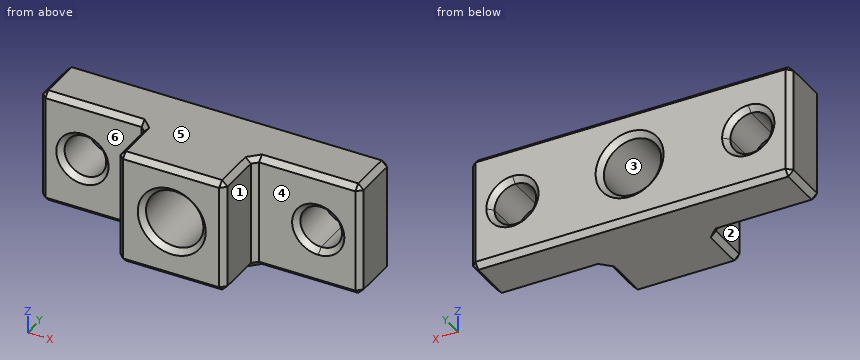
```python
from build123d import *

# Parameters (mm, degrees)
F0_W      = 30.2609670907
F0_H      = 10.7729053125
F1_DEPTH  = 10
F2_W      = 10.0509477779
F2_H      = 10.7729053125
F3_DEPTH  = 5
F4_W      = 10.0912228227
F4_H      = 10.7729053125
F5_DEPTH  = 5
F6_W      = 10.084872134
F6_H      = 10.7729053125
F7_DEPTH  = 5
F8_R      = 2.7105464677
F9_DEPTH  = 25
F11_DEPTH = 25
F13_DEPTH = 25
F14_SIZE  = 0.5


with BuildPart() as f1:
    # F0 (on Front) → F1 (new body)
    with BuildSketch(Plane.XZ):
        with Locations((15.1304835454, -5.3864526562)):
            Rectangle(F0_W, F0_H)
    extrude(amount=F1_DEPTH)

    # F2 (on face) → F3 (join)
    with BuildSketch(Plane.XZ.offset(10)):
        with Locations((5.025473889, -5.3864526562)):
            Rectangle(F2_W, F2_H)
    extrude(amount=-F3_DEPTH)

    # F4 (on face) → F5 (cut)
    with BuildSketch(Plane.XZ.offset(10)):
        with Locations((5.0456114113, -5.3864526562)):
            Rectangle(F4_W, F4_H)
    extrude(amount=-F5_DEPTH, mode=Mode.SUBTRACT)

    # F6 (on face) → F7 (cut)
    with BuildSketch(Plane.XZ.offset(10)):
        with Locations((25.2185310237, -5.3864526562)):
            Rectangle(F6_W, F6_H)
    extrude(amount=-F7_DEPTH, mode=Mode.SUBTRACT)

    # F8 (on face) → F9 (cut)
    with BuildSketch(Plane.XZ.offset(10)):
        with Locations((15.200487338, -5.2238842472)):
            Circle(F8_R)
    extrude(amount=-F9_DEPTH, mode=Mode.SUBTRACT)

    # F10 (on face) → F11 (cut)
    with BuildSketch(Plane.XZ.offset(5)):
        with BuildLine():
            ThreePointArc((5.9674986844, -5.3864526562), (5.3912316617, -3.9952209945), (4, -3.4189539719))
            Line((4, -3.4189539719), (4, -7.3539513406))
            ThreePointArc((4, -7.3539513406), (5.3912316617, -6.7776843179), (5.9674986844, -5.3864526562))
        make_face()
        with BuildLine():
            Line((4, -7.3539513406), (4, -3.4189539719))
            ThreePointArc((4, -3.4189539719), (2.0325013156, -5.3864526562), (4, -7.3539513406))
        make_face()
    extrude(amount=-F11_DEPTH, mode=Mode.SUBTRACT)

    # F12 (on face) → F13 (cut)
    with BuildSketch(Plane.XZ.offset(5)):
        with BuildLine():
            ThreePointArc((28.2237478891, -5.3864526562), (27.6488627033, -3.9985570437), (26.2609670907, -3.4236718578))
            Line((26.2609670907, -3.4236718578), (26.2609670907, -7.3492334546))
            ThreePointArc((26.2609670907, -7.3492334546), (27.6488627033, -6.7743482688), (28.2237478891, -5.3864526562))
        make_face()
        with BuildLine():
            Line((26.2609670907, -7.3492334546), (26.2609670907, -3.4236718578))
            ThreePointArc((26.2609670907, -3.4236718578), (24.2981862923, -5.3864526562), (26.2609670907, -7.3492334546))
        make_face()
    extrude(amount=-F13_DEPTH, mode=Mode.SUBTRACT)

    # F14
    f14_edges = [f1.edges().sort_by_distance(p)[0] for p in [
        (12.489941, -10, -5.223884),
        (24.298186, -5, -5.386453),
        (2.032501, -5, -5.386453),
        (10.091223, -7.5, -10.772905),
        (10.091223, -7.5, 0),
        (10.091223, -10, -5.386453),
        (10.091223, -5, -5.386453),
        (15.130484, 0, -10.772905),
        (30.260967, -2.5, -10.772905),
        (25.218531, -5, -10.772905),
        (20.176095, -7.5, -10.772905),
        (15.133659, -10, -10.772905),
        (5.045611, -5, -10.772905),
        (0, -2.5, -10.772905),
        (0, 0, -5.386453),
        (0, -5, -5.386453),
        (0, -2.5, 0),
        (15.130484, 0, 0),
        (5.045611, -5, 0),
        (15.133659, -10, 0),
        (20.176095, -7.5, 0),
        (25.218531, -5, 0),
        (30.260967, -2.5, 0),
        (20.176095, -10, -5.386453),
        (20.176095, -5, -5.386453),
        (30.260967, 0, -5.386453),
        (30.260967, -5, -5.386453),
        (2.032501, 0, -5.386453),
        (24.298186, 0, -5.386453),
        (12.489941, 0, -5.223884),
    ]]
    chamfer(f14_edges, length=F14_SIZE)


solid = f1.part
```
Part model, mm, in its own coordinate system. Face numbers are marked on the shaded views. A direction names the side the tool comes from. Give positions to 0.01 mm unless a question says otherwise; leave off trailing zeros. Order: outer loops, then holes, each group sorted by start corner. A loop starts at its lowest first (then second) coordinate and runs counter-clockwise, first axis right, second up. Notation, with made-up numbers: (28, 84.25) - (41, 84.25) arc R14 ccw to (41, 90.25) - close; hole circle Ø11 at (-18, -2). An arc over 180 degrees is marked (long way). Use one line per item in the form item = value.
Item 1: Pin check, flat tips, straight feed: pin 1 Ø1.5 at (x, z) = (20.5, -9) entering from -Y; pin 2 Ø3 at (x, z) = (4, -5.39) entering from -Y; pin 3 Ø2 at (y, z) = (-7.5, -7.5) entering from +X; pin 4 Ø1.5 at (y, z) = (-7, -2) entering from -X. Stop position of each tip, or through.
Solution:
pin_1 = -9.93
pin_2 = through
pin_3 = 20.18
pin_4 = 10.09
Item 2: Slice it at B-B on z = -9. Give the cut face in (x, y).
Solution:
outline = (0, -4.5) - (0.5, -5) - (9.59, -5) - (10.09, -5.5) - (10.09, -9.5) - (10.59, -10) - (19.68, -10) - (20.18, -9.5) - (20.18, -5.5) - (20.68, -5) - (29.76, -5) - (30.26, -4.5) - (30.26, -0.5) - (29.76, 0) - (0.5, 0) - (0, -0.5) - close
Item 3: Two-plate mould, pull along X, no slides. Class the marked faces 1, 2 and 3: released by +X, released by -X, zero draft, split by the parting line, or undercut.
Solution:
face_1 = released by +X
face_2 = released by -X
face_3 = undercut
Item 4: Which spindle directions (+Z, -Z, +X, -X, +Y, -Y) get a long thin tool onto all of the face, cutting with end or side? Do the marked faces 4, 5 and 6. Say none if no direction does.
Solution:
face_4 = +Z, -Z, +X, -Y
face_5 = +Z, +X, -X, +Y, -Y
face_6 = +Z, -Z, -X, -Y
Item 5: Probe probe 1 along Z at (x, y) = (4, -2.3); probe 2 along X at (y, z) = (-2.25, -4.25); probe 3 along X at (y, z) = (-1.5, -4). List the from-to ranges inside material, lowest first. Write a range as from..to.
Solution:
probe_1 = -10.77..-7.35, -3.42..0
probe_2 = 0..2.39, 5.61..12.67, 17.73..24.66, 27.86..30.26
probe_3 = 0..2.6, 5.4..12.78, 17.62..24.87, 27.65..30.26
Item 6: Slice it at C-C on y = -1. Give the cut face in (x, z) (1 decimal), and give its area (3 significant figures).
Solution:
outline = (0, -10.3) - (0.5, -10.8) - (29.8, -10.8) - (30.3, -10.3) - (30.3, -0.5) - (29.8, 0) - (0.5, 0) - (0, -0.5) - close; hole circle Ø3.9 at (4, -5.4); hole circle Ø5.4 at (15.2, -5.2); hole circle Ø3.9 at (26.3, -5.4)
area = 278 mm2
Item 7: Slice it at D-D on z = -4.5. Count the separate pieces of the cut face and the enclosed holes in it, and give its area (3 significant figures).
Solution:
separate_pieces = 4
enclosed_holes = 0
area = 112 mm2
Item 8: Slice it at A-A on y = -7.75. Give the cut face in (x, z).
Solution:
outline = (10.09, -10.27) - (10.59, -10.77) - (19.68, -10.77) - (20.18, -10.27) - (20.18, -0.5) - (19.68, 0) - (10.59, 0) - (10.09, -0.5) - close; hole circle Ø5.42 at (15.2, -5.22)
